The model under review builds one solid part; all positions refer to its coordinate system, in mm. A direction names the side the tool comes from. Round coordinates to 2 decimals unless told otherwise and drop trailing zeros. Loops run counter-clockwise (first coordinate to the right, second up) from the corner with the lowest first, then second, coordinate; pieces in that order, holes last. Notation, with made-up numbers: (78.25, -33.5) - (114.25, -33.5) arc R24 cw to (114.25, 3.5) - close; hole circle Ø3 at (33, 42.25). An arc over 180 degrees is marked (long way). Answer as CSV lines item,"result".
Autodesk Fusion 360 part; units mm, degrees
sketch "Esquisse1" plane through (0, 0, 0) normal (1, 0, 0) x (0, 1, 0)
  line L0 (0, 0) -> (-250, 0) construction
  line L1 (-250, 0) -> (-250, 150) construction
  line L2 (-220, 150) -> (0, 150) construction
  line L3 (0, 150) -> (0, 0) construction
  line L4 (0, 0) -> (0, 39.75)
  line L5 (-10, 39.75) -> (0, 39.75)
  line L6 (-10, 39.75) -> (-10, 60.25)
  line L7 (-10, 60.25) -> (0, 60.25)
  line L8 (0, 60.25) -> (0, 89.75)
  line L9 (-10, 89.75) -> (-10, 110.25)
  line L10 (-10, 110.25) -> (0, 110.25)
  line L11 (-10, 89.75) -> (0, 89.75)
  line L12 (0, 110.25) -> (0, 125)
  line L13 (-13.3649, 150) -> (-250, 150) construction
  line L14 (11, 150) -> (1, 150) construction
  line L15 (1, 150) -> (1, 140) construction
  line L16 (1, 140) -> (11, 140) construction
  line L17 (11, 140) -> (11, 150) construction
  line L18 (11, 150) -> (1, 140) construction
  line L19 (1, 150) -> (11, 140) construction
  arc A0 (6, 125) -> (-13.3649, 150) centre (6, 145) ccw
  line L20 (-13.3649, 150) -> (-220, 150)
  line L21 (-250, 140) -> (-250, 110.5)
  line L22 (-250, 110.5) -> (-240, 110.5)
  line L23 (-240, 110.5) -> (-240, 90)
  line L24 (-240, 90) -> (-250, 90)
  line L25 (-250, 90) -> (-250, 60.5)
  line L26 (-250, 60.5) -> (-240, 60.5)
  line L27 (-240, 60.5) -> (-240, 40)
  line L28 (-240, 40) -> (-250, 40)
  line L29 (-250, 40) -> (-250, 0)
  line L30 (-250, 0) -> (-150.25, 0)
  line L31 (-150.25, 0) -> (-150.25, 10)
  line L32 (-150.25, 10) -> (-99.75, 10)
  line L33 (-99.75, 10) -> (-99.75, 0)
  line L34 (-99.75, 0) -> (0, 0)
  line L35 (-125, 150) -> (-125, 10) construction
  line L36 (-250, 75) -> (0, 75) construction
  circle A1 centre (6, 145) radius 7.5
  circle A2 centre (6, 145) radius 7.0711 construction
  line L37 (-125, 150) -> (-125, 0) construction
  line L38 (-225, 145) -> (-225, 140)
  line L39 (-225, 140) -> (-250, 140)
  line L40 (0, 140) -> (-250, 140) construction
  line L41 (0, 125) -> (6, 125)
  arc A3 (6, 125) -> (0, 125.9212) centre (6, 145) ccw construction
  arc A4 (0, 125.9212) -> (6, 125) centre (6, 145) ccw construction
  arc A5 (-220, 150) -> (-225, 145) centre (-220, 145) ccw
  point P0 (6, 145)
  point P1 (-10, 100)
  point P2 (-10, 50)
  dimension "d1" = 250
  dimension "d2" = 150
  dimension "d4" = 20.5
  dimension "d7" = 10
  dimension "d8" = 40
  dimension "d11" = 10
  dimension "d12" = 10
  dimension "d13" = 40
  dimension "d29" = 50.5
  dimension "d30" = 10
  dimension "d36" = 140
  dimension "d37" = 10
  dimension "d38" = 1
  dimension "d40" = 5
  dimension "d41" = 50
  dimension "d42" = 15
  dimension "d43" = 25
extrude "Extrusion1" add sketch "Esquisse1" along normal blind 10
sketch "Esquisse2" plane through (10, 0, 0) normal (1, 0, 0) x (0, 1, 0)
  circle A0 centre (6, 145) radius 7.5
  line L0 (-250, 140) -> (-250, 110.5)
  line L1 (-250, 110.5) -> (-240, 110.5)
  line L2 (-240, 110.5) -> (-240, 90)
  line L3 (-240, 90) -> (-250, 90)
  line L4 (-250, 90) -> (-250, 60.5)
  line L5 (-250, 60.5) -> (-240, 60.5)
  line L6 (-240, 60.5) -> (-240, 40)
  line L7 (-240, 40) -> (-250, 40)
  line L8 (-250, 40) -> (-250, 0)
  line L9 (-250, 0) -> (-150.25, 0)
  line L10 (-150.25, 0) -> (-150.25, 10)
  line L11 (-150.25, 10) -> (-99.75, 10)
  line L12 (-99.75, 10) -> (-99.75, 0)
  line L13 (-99.75, 0) -> (0, 0)
  line L14 (0, 0) -> (0, 39.75)
  line L15 (0, 39.75) -> (-10, 39.75)
  line L16 (-10, 39.75) -> (-10, 60.25)
  line L17 (-10, 60.25) -> (0, 60.25)
  line L18 (0, 60.25) -> (0, 89.75)
  line L19 (0, 89.75) -> (-10, 89.75)
  line L20 (-10, 89.75) -> (-10, 110.25)
  line L21 (-10, 110.25) -> (0, 110.25)
  line L22 (0, 110.25) -> (0, 125)
  arc A1 (6, 125) -> (-13.3649, 150) centre (6, 145) ccw
  line L23 (-13.3649, 150) -> (-220, 150)
  line L24 (-250, 12.7) -> (0, 12.7) construction
  circle A2 centre (-215, 12.7) radius 2.5
  circle A3 centre (-190, 12.7) radius 2.5
  circle A4 centre (-165, 12.7) radius 2.5
  line L25 (-250, 10.2) -> (0, 10.2) construction
  line L26 (-125, 140) -> (-125, 10)
  circle A5 centre (-35, 12.7) radius 2.5
  circle A6 centre (-85, 12.7) radius 2.5
  circle A7 centre (-60, 12.7) radius 2.5
  line L27 (-225, 145) -> (-225, 140)
  line L28 (-225, 140) -> (-250, 140)
  line L29 (0, 125) -> (6, 125)
  arc A8 (-220, 150) -> (-225, 145) centre (-220, 145) ccw
  point P0 (0, 12.7)
  point P1 (0, 10.2)
  dimension "d22" = 5
  dimension "d24" = 0.2
  dimension "d25" = 25
  dimension "d26" = 25
  dimension "d27" = 35
extrude "Extrusion2" cut sketch "Esquisse2" against normal through all contours A2 | A3 | A4 | A5 | A6 | A7
1. Wall thickness on probe 1 along Z at (x, y) = (4.5, -165); probe 2 along Z at (x, y) = (3, 6); probe 3 along Z at (x, y) = (5.25, -236): over which ranges is each line inside the solid? List them lowest first.
Numbers:
probe 1,"z = 0 to 10.2, 15.2 to 150"
probe 2,"z = 125 to 137.5, 152.5 to 165"
probe 3,"z = 0 to 140"
2. Draft analysis for pull direction Y (two halves, no side actions). For faces 1 (the face through (4.93, 21.421, 157.735)), 2 (the face through (5, -5, 89.75)), 3 (the face through (4.93, 5.024, 137.564)), 4 (the face through (5.07, -187.615, 13.451)), state which applies: +Y half, -Y half, draft (parallel to the pull), parting line (faces both ways), or undercut.
Numbers:
face 1,"parting line"
face 2,"draft"
face 3,"undercut"
face 4,"undercut"
3. Take a section at C-C (y = -132). State the section outline as (x, z) points.
Numbers:
outline,"(0, 10) - (10, 10) - (10, 150) - (0, 150) - close"
4. Clearance check with flat-ended pins moving along their axes: pin 1 (4 mm diameter, centred on y = -45.5, z = 124, fed in from -X); pin 2 (3 mm diameter, centred on x = 2.5, y = -68.5, fed in from +Z); pin 3 (2.5 mm diameter, centred on x = 6.5, z = 143, fed in from -Y); pin 4 (3 mm diameter, centred on x = 7, z = 53, fed in from -Y). State where each tip first meets the part, or that it passes through.
Numbers:
pin 1,"stops at x = 0"
pin 2,"stops at z = 150"
pin 3,"stops at y = -225"
pin 4,"stops at y = -240"
5. Take a section at B-B (z = 56.5). State the section outline as (x, y) points, plus the area to 3 significant figures.
Numbers:
outline,"(0, -240) - (10, -240) - (10, -10) - (0, -10) - close"
area,"2,300 mm²"
6. Take a section at A-A (x = 2.75). State how many separate pieces and enclosed holes the cut face has, plus the area to 3 significant figures.
Numbers:
separate pieces,"1"
enclosed holes,"7"
area,"36,600 mm²"
7. Tool access review of faces 5 (the face through (5, -115, 150)), 6 (the face through (5, -245, 60.5)), 7 (the face through (5, 0, 118)): name each direction out of +Z, -Z, +X, -X, +Y, -Y from which nothing blocks a thin tool from reaching the whole face with its end or side.
Numbers:
face 5,"+Z, +X, -X, -Y"
face 6,"+X, -X, -Y"
face 7,"-Z, +X, -X, +Y"
